Could you check a few things on this drawing? It's one solid part, dimensions in mm from its lowest x, y, z. A direction names the side the tool comes from. Give positions to 0.01 mm unless a question says otherwise; leave off trailing zeros. Write each loop counter-clockwise with the first axis right and the second up, starting at its lowest first coordinate (ties: lowest second). Pieces come first, ordered by that corner, then holes. Notation, with made-up numbers: M 67,-36 L 88,-36 A8 cw 88,-32 Z; hole C 65,-37 d1. An arc over 180 degrees is marked long. Write each question's results on one line, items separated by ' | '.
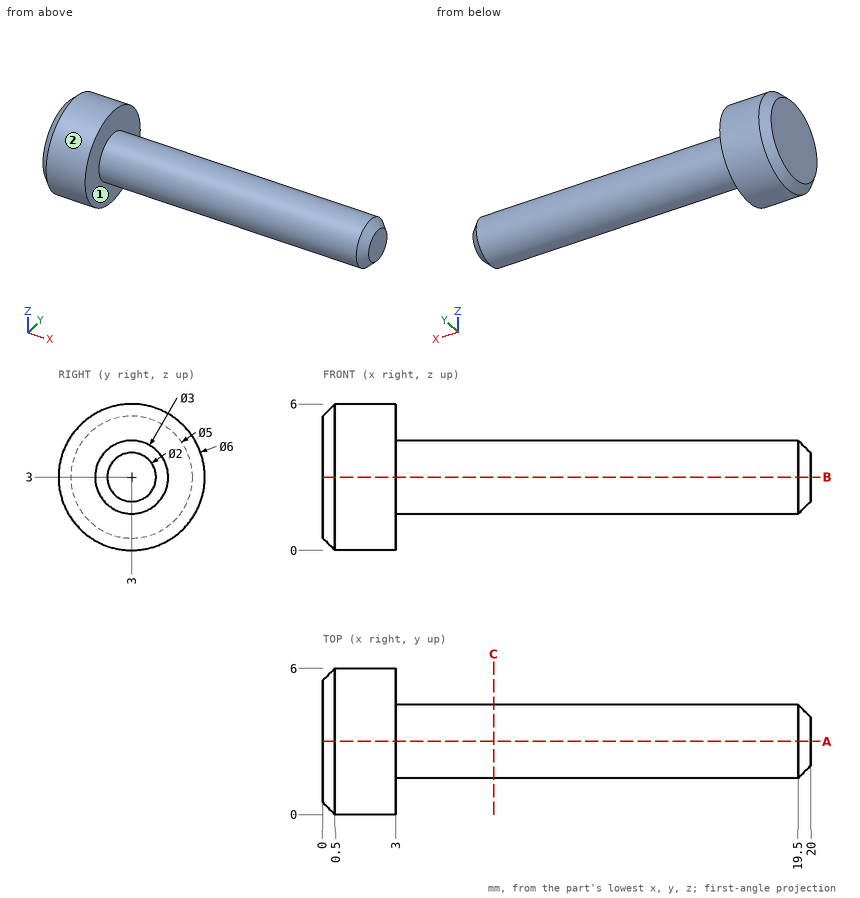
Item 1: I want a section at C-C, the plane x = 7. Please give me the cut outline in (y, z).
Geometry says:
outline: C 3,3 d3
Item 2: I want a section at A-A, the plane y = 3. Please give me the cut outline in (x, z), and give its area (3 significant figures).
Geometry says:
outline: M 0,0.5 L 0.5,0 L 3,0 L 3,1.5 L 19.5,1.5 L 20,2 L 20,4 L 19.5,4.5 L 3,4.5 L 3,6 L 0.5,6 L 0,5.5 Z | area: 68.5 mm2
Item 3: For the marked faces 1 and 2, which set-ups out of +Z, -Z, +X, -X, +Y, -Y let a thin tool reach every point of the face, with its end or its side?
Geometry says:
face 1: +X | face 2: +X, -X
Item 4: I'm going to push flat-ended pins straight in: pin 1 (2 mm diameter, centred on x = 3, y = 4.5, fed in from -Z); pin 2 (3 mm diameter, centred on y = 4, z = 4, fed in from +X); pin 3 (1 mm diameter, centred on x = 8, z = 3.5, fed in from -Y); pin 4 (1 mm diameter, centred on x = 15.5, z = 2, fed in from -Y). Where does each tip first touch, or does it pass through?
Geometry says:
pin 1: stops at z = 0.04 | pin 2: stops at x = 20 | pin 3: stops at y = 1.5 | pin 4: stops at y = 1.59
Item 5: If I drill on line 1 (X direction, y = 3.55, z = 4.8); line 2 (Z direction, x = 1.75, y = 0.75); line 3 (Y direction, x = 15, z = 2.4), over which ranges is the centre line in solid material (lowest first)? Write a range as from..to.
Geometry says:
line 1: x = 0..3 | line 2: z = 1.02..4.98 | line 3: y = 1.63..4.37
